Can you work these out from the model? Positions are in its coordinate system, mm. A direction names the side the tool comes from. Coordinates: 2 decimals unless noted, no trailing zeros. Order: outer loops, then holes, each group sorted by start corner. A loop starts at its lowest first (then second) coordinate and runs counter-clockwise, first axis right, second up. Notation, with made-up numbers: (25.5, 28.25) - (53.5, 28.25) arc R11 ccw to (53.5, 48.25) - close; hole circle Ø1 at (50.25, -0.5). An arc over 180 degrees is marked (long way). Use a Markdown table: item, result. Add a question column.
(1) For pin 1 Ø2.5 at (x, y) = (47.01, 31.34) entering from -Z; pin 2 Ø3.5 at (x, y) = (-47.01, -31.34) entering from -Z; pin 3 Ø3 at (x, z) = (27.5, 4) entering from +Y; pin 4 Ø3 at (y, z) = (40.5, 4) entering from -X, each with a flat end and sliding along its axis, tell me the tip position at first contact or that it passes through.
(2) We'd pull the mould along Y, two halves only. Please class faces 1 (the flat face through (-27, -13, 0)), 2 (the cylindrical face through (50.174, -34.714, 5.817)), 3 (the flat face through (-48.3, 30, 4)): pulls with the +Y half, pulls with the -Y half, needs draft (parallel to the pull), parting line crosses it, or undercut.
(3) On a 3-axis mill with a long thin cutter (end or side, diameter ignored), from which of +Z, -Z, +X, -X, +Y, -Y can I reach the whole of each face in a straight line? I mean faces 4 (the flat face through (-23, -46, 4.6)), 5 (the flat face through (51.6, 3.1, 7)), 6 (the cylindrical face through (-44.15, 30.44, 1.97)). Say none if no direction works.
(4) If I drill on L1, parallel to Y at x = -47.5, z = 3.25; L2, parallel to X at y = 5.5, z = 6; L3, parallel to X at y = 34, z = 1.5, over which ranges is the centre line in solid material (lowest first)? Write a range as [from, to].
(5) I want a section at B-B (y = 53). List the corners of the cut face in (x, z) for me.
Autodesk Inventor part; units mm, degrees
ref_plane "YZ Plane" through (0, 0, 0) normal (1, 0, 0) x (0, 1, 0)
ref_plane "XZ Plane" through (0, 0, 0) normal (0, 1, 0) x (-1, 0, 0)
ref_plane "XY Plane" through (0, 0, 0) normal (0, 0, 1) x (1, 0, 0)
sketch "Sketch1" plane through (0, 0, 0) normal (0, 0, 1) x (1, 0, 0)
  circle A0 centre (-47.0107, -31.3407) radius 4.8
  arc A1 (51.632, -32.6385) -> (49.9861, -35.1073) centre (47.0107, -31.3407) ccw
  arc A2 (51.632, -32.6385) -> (51.632, 32.6385) centre (0, 0) ccw
  arc A3 (49.9861, 35.1073) -> (51.632, 32.6385) centre (47.0107, 31.3407) ccw
  arc A4 (49.9861, 35.1073) -> (-42.369, 44) centre (0, 0) ccw
  line L0 (-42.369, 44) -> (-62, 44)
  line L1 (-62, 44) -> (-64, 42)
  line L2 (-64, 42) -> (-64, 0.1)
  arc A5 (0, -61.083) -> (49.9861, -35.1073) centre (0, 0) ccw
  circle A6 centre (0, 0) radius 48
  circle A7 centre (-58, 38) radius 3.825
  circle A8 centre (-47.0107, 31.3407) radius 4.8
  line L3 (0, 0) -> (-74.8823, 0)
  circle A9 centre (-58, -38) radius 3.825
  line L4 (-42.369, -44) -> (-62, -44)
  arc A10 (-42.369, -44) -> (49.9861, -35.1073) centre (0, 0) ccw
  line L5 (-62, -44) -> (-64, -42)
  line L6 (-64, -42) -> (-64, 0.1)
extrude "Extrusion1" add sketch "Sketch1" along normal blind 4.8
sketch "Sketch5" plane through (0, 0, 4.8) normal (0, 0, 1) x (1, 0, 0)
  circle A0 centre (0, 0) radius 48
  circle A1 centre (-47.0107, 31.3407) radius 4.8
  circle A2 centre (0, 0) radius 61.5
  arc A3 (49.9861, 35.1073) -> (51.632, 32.6385) centre (47.0107, 31.3407) ccw
  circle A4 centre (47.0107, 31.3407) radius 1.6
  arc A5 (51.632, -32.6385) -> (49.9861, -35.1073) centre (47.0107, -31.3407) ccw
  circle A6 centre (47.0107, -31.3407) radius 1.6
  circle A7 centre (-47.0107, -31.3407) radius 4.8
  circle A8 centre (-47.0107, -31.3407) radius 1.6
  circle A9 centre (-47.0107, 31.3407) radius 4.8
  circle A10 centre (-47.0107, 31.3407) radius 1.6
  dimension "d14" = 123
  dimension "d41" = 3.2
  dimension "d42" = 3.2
  dimension "d43" = 3.2
  dimension "d44" = 3.2
extrude "Extrusion5" add sketch "Sketch5" against normal up to surface (4.8 mm away) contours A1 | A2 | A7
sketch "Sketch8" plane through (0, 0, 0) normal (0, 0, -1) x (-1, 0, 0)
  circle A0 centre (0, 0) radius 48
  circle A1 centre (0, 0) radius 29
  dimension "d30" = 58
extrude "Extrusion8" add sketch "Sketch8" against normal up to surface (4.8 mm away)
sketch "Sketch9" plane through (0, 0, 0) normal (0, 0, -1) x (-1, 0, 0)
  circle A0 centre (0, 0) radius 29
  circle A1 centre (0, 0) radius 27.5
  dimension "d33" = 1.5
extrude "Extrusion9" add sketch "Sketch9" against normal blind 1
chamfer "Chamfer3" distance 1 angle 45 1 edges at (29, 0, 1)
sketch "Sketch10" plane through (0, 0, 4.8) normal (0, 0, 1) x (1, 0, 0)
  circle A0 centre (0, 0) radius 29
  circle A1 centre (-58, 38) radius 3.825
  arc A2 (-42.968, -44) -> (-42.968, 44) centre (0, 0) ccw
  line L0 (-42.968, 44) -> (-62, 44)
  line L1 (-62, 44) -> (-64, 42)
  line L2 (-64, 42) -> (-64, -42)
  circle A3 centre (47.0107, 31.3407) radius 1.6
  circle A4 centre (47.0107, -31.3407) radius 1.6
  circle A5 centre (-47.0107, -31.3407) radius 1.6
  circle A6 centre (-47.0107, 31.3407) radius 1.6
  line L3 (-64, -42) -> (-62, -44)
  line L4 (-62, -44) -> (-42.968, -44)
  circle A7 centre (-58, -38) radius 3.825
extrude "Extrusion10" add sketch "Sketch10" along normal blind 2.2
sketch "Sketch11" plane through (0, 0, 0) normal (0, 0, -1) x (-1, 0, 0)
  circle A0 centre (-47.0107, -31.3407) radius 1.6
  circle A1 centre (-47.0107, -31.3407) radius 3
  circle A2 centre (-47.0107, 31.3407) radius 1.6
  circle A3 centre (-47.0107, 31.3407) radius 3
  circle A4 centre (47.0107, 31.3407) radius 1.6
  circle A5 centre (47.0107, 31.3407) radius 3
  circle A6 centre (47.0107, -31.3407) radius 1.6
  circle A7 centre (47.0107, -31.3407) radius 3
  point P0 (0, 0)
  dimension "d45" = 6
  dimension "d46" = 6
  dimension "d47" = 6
  dimension "d48" = 6
extrude "Extrusion11" cut sketch "Sketch11" against normal blind 4 contours A1 | A3 | A5 | A6 | A7
sketch "Sketch12" plane through (0, 0, 7) normal (0, 0, 1) x (1, 0, 0)
  circle A0 centre (0, 0) radius 48
  circle A1 centre (0, 0) radius 51
  dimension "d51" = 96
  dimension "d52" = 3
extrude "Extrusion12" cut sketch "Sketch12" against normal blind 1.5
chamfer "Chamfer4" distance 1.5 angle 45 2 edges at (-51, 0, 5.5) (-48, 0, 5.5)
sketch "Sketch17" plane through (0, 0, 7) normal (0, 0, 1) x (1, 0, 0)
  circle A0 centre (0, 0) radius 61.5
  circle A1 centre (0, 0) radius 96.3014
  point P0 (-42.968, 44)
extrude "Extrusion15" cut sketch "Sketch17" against normal through all
sketch "Sketch19" plane through (0, 0, 0) normal (0, 0, -1) x (-1, 0, 0)
  circle A0 centre (-47.0107, -31.3407) radius 3
  line L0 (0, 0) -> (-47.0107, -31.3407)
  line L1 (-47.0107, -31.3407) -> (-60.1837, -40.1228)
  circle A1 centre (0, 0) radius 65
  circle A2 centre (0, 0) radius 61.5
  circle A3 centre (-54.0831, -36.0557) radius 2.05
  circle A4 centre (-54.0831, -36.0557) radius 4
  line L2 (-54.8676, -39.978) -> (-36.9294, -43.5656)
  line L3 (-58.0055, -35.2712) -> (-54.4179, -17.333)
  point P0 (-44.9634, -41.9588)
  point P1 (-56.0247, -25.367)
  point P2 (-58.0055, -35.2712)
  dimension "d67" = 130
  dimension "d69" = 8
  dimension "d68" = 4.1
  dimension "d70" = 45
extrude "Extrusion16" add sketch "Sketch19" against normal up to surface (7 mm away) contours A2 A4 A1 A3 L1 | L1 A3 A1 A4 A2 | A2 L2 A1 A4 | A4 A1 L3 A2 | A4 L3 A1 | A1 A3 L1 A4 | L2 A4 A1 | A4 L1 A3 A1
sketch "Sketch20" plane through (0, 0, 7) normal (0, 0, 1) x (1, 0, 0)
  arc A0 (33.0898, 38.808) -> (-18.5896, 47.4913) centre (0, 0) ccw
  line L0 (45.7919, 36.955) -> (33.0898, 38.808)
  arc A1 (51.7244, 28.0563) -> (45.7919, 36.955) centre (44.9997, 30) ccw
  line L1 (48.5496, 15.6186) -> (51.7244, 28.0563)
  arc A2 (48.5496, -15.6186) -> (48.5496, 15.6186) centre (0, 0) ccw
  line L2 (51.7244, -28.0563) -> (48.5496, -15.6186)
  arc A3 (45.7919, -36.955) -> (51.7244, -28.0563) centre (44.9997, -30) ccw
  line L3 (33.0898, -38.808) -> (45.7919, -36.955)
  arc A4 (-18.5896, -47.4913) -> (33.0898, -38.808) centre (0, 0) ccw
  line L4 (-33.7876, -44) -> (-18.5896, -47.4913)
  line L5 (-62, -44) -> (-33.7876, -44)
  line L6 (-64, -42) -> (-62, -44)
  line L7 (-64, 42) -> (-64, -42)
  line L8 (-62, 44) -> (-64, 42)
  line L9 (-33.7876, 44) -> (-62, 44)
  line L10 (-18.5896, 47.4913) -> (-33.7876, 44)
  circle A5 centre (0, 0) radius 88.8325
extrude "Extrusion17" cut sketch "Sketch20" against normal blind 2.4
sketch "Sketch21" plane through (0, 0, 0) normal (0, 0, -1) x (-1, 0, 0)
  circle A0 centre (0, 0) radius 78.6238
  circle A1 centre (0, 0) radius 61.5
extrude "Extrusion18" cut sketch "Sketch21" against normal through all
sketch "Sketch22" plane through (0, 0, 0) normal (0, 0, -1) x (-1, 0, 0)
  circle A0 centre (0, 0) radius 61.5
  circle A1 centre (0, 0) radius 27.5
  circle A2 centre (0, 0) radius 62.5
  dimension "d77" = 1
extrude "Extrusion19" add sketch "Sketch22" against normal up to surface (4.6 mm away) contours A2
sketch "Sketch23" plane through (0, 0, 7) normal (0, 0, 1) x (1, 0, 0)
  circle A0 centre (47.0107, 31.3407) radius 1.6
  line L0 (48.5496, 15.6186) -> (51.7244, 28.0563)
  arc A1 (51.7244, 28.0563) -> (45.7919, 36.955) centre (44.9997, 30) ccw
  line L1 (45.7919, 36.955) -> (33.0898, 38.808)
  arc A2 (48.5496, 15.6186) -> (33.0898, 38.808) centre (0, 0) ccw
  line L2 (51.7244, -28.0563) -> (48.5496, -15.6186)
  arc A3 (33.0898, -38.808) -> (48.5496, -15.6186) centre (0, 0) ccw
  line L3 (33.0898, -38.808) -> (45.7919, -36.955)
  arc A4 (45.7919, -36.955) -> (51.7244, -28.0563) centre (44.9997, -30) ccw
  circle A5 centre (47.0107, -31.3407) radius 1.6
  arc A6 (48.5496, -15.6186) -> (48.5496, 15.6186) centre (0, 0) ccw
  line L4 (51.9997, 39.8529) -> (51.9997, -52.1761)
  point P0 (51.9997, -30)
  point P1 (51.9997, 30)
extrude "Extrusion20" add sketch "Sketch23" against normal up to surface (2.4 mm away) contours L0 A1 L4 A4 L2 A6
sketch "Sketch24" plane through (0, 0, 7) normal (0, 0, 1) x (1, 0, 0)
  line L0 (0, -84.8798) -> (-71.6508, -84.8798)
  line L1 (-71.6508, -84.8798) -> (-71.6508, 87.4797)
  line L2 (-71.6508, 87.4797) -> (0, 87.4797)
  line L3 (0, 87.4797) -> (0, -84.8798)
  point P0 (0, 0)
extrude "Extrusion21" cut sketch "Sketch24" along normal through all both and the other way through all
mirror "Mirror1" about plane through (0, -84.8798, 7) normal (-1, 0, 0)
properties part number "frame_rring2"
Answers follow:
| question | item | result |
|---|---|---|
| 1 | pin 1 | passes through |
| 1 | pin 2 | stops at z = 4 |
| 1 | pin 3 | stops at y = 56.84 |
| 1 | pin 4 | stops at x = -48.84 |
| 2 | face 1 | needs draft |
| 2 | face 2 | pulls with the -Y half |
| 2 | face 3 | undercut |
| 3 | face 4 | +Z |
| 3 | face 5 | +Z, +X, -X, +Y, -Y |
| 3 | face 6 | -Z |
| 4 | L1 | y = [-40.62, -34.3], [-28.38, 28.38], [34.3, 40.62] |
| 4 | L2 | x = [-52, -49.7], [-48.69, -28.47], [28.47, 48.69], [49.7, 52] |
| 4 | L3 | x = [-52.44, -48.4], [-45.62, 45.62], [48.4, 52.44] |
| 5 | outline | (-33.12, 0) - (33.12, 0) - (33.12, 4.6) - (-33.12, 4.6) - close |
